Check sheet for the modelled part. Datum: model origin and axes. Units: mm. A direction names the side the tool comes from. Give positions to 0.01 mm unless a question says otherwise; leave off trailing zeros. Write each loop counter-clockwise with the first axis right and the second up, starting at its lowest first coordinate (ties: lowest second). Pieces come first, ordered by that corner, then holes. Notation, with made-up numbers: M 76,41 L 117,41 A36 cw 117,77 Z; hole C -34,10.25 d8. An arc over 180 degrees is marked long. Use CSV: the item, a comma, the result in double quotes. Start each with the question number.
1. Cross-section at A-A, the plane x = 16. Enter the section's corners in (y, z).
2. Mould release check, pull along Z, two halves, no side actions. Record for faces 1 (the face through (0, -6, 8)), 2 (the face through (19.699, 5.803, 0.285)), 3 (the face through (14.4, 5.8, 3.07)): +Z half, -Z half, draft (parallel to the pull), parting line (faces both ways), or undercut.
3. Depth check by flat-ended pin: P1, Ø5, axis at x = 5.5, y = 1.5, coming from the -Z side; P2, Ø4, axis at x = 16, z = 3, coming from the -Y side. Enter the tip coordinate at first touch or a pass-through.
4. Scan lines: line 1 (Y direction, x = -4.5, z = 8.5); line 2 (Z direction, x = 16, y = 5.8); line 3 (Z direction, x = 2, y = -0.75). Record each from-to range of solid material in increasing order.
5. Cross-section at D-D, the plane x = 6.5. Enter the section's corners in (y, z), and give its area (3 significant figures).
6. Access from +Z, -Z, +X, -X, +Y, -Y to the whole of each face (thin tool, end or side, straight path). Record for faces 4 (the face through (0, 0, 15.6)), 5 (the face through (-19.715, 5.803, 0.301)).
7. Cross-section at C-C, the plane z = 11. Enter the section's corners in (x, y), and give its area (3 significant figures).
8. Cross-section at B-B, the plane z = 3. Enter the section's corners in (x, y), and give its area (3 significant figures).
from build123d import *

# Parameters (mm, degrees)
SKETCH1_W           = 40
SKETCH1_H           = 12
BOSS_EXTRUDE1_DEPTH = 16
SKETCH2_R           = 1.6
SKETCH2_W           = 12
SKETCH2_H           = 0.6
CUT_EXTRUDE1_DEPTH  = 13
SKETCH3_W           = 15.6
SKETCH3_H           = 11.2
CUT_EXTRUDE2_DEPTH  = 41
FILLET1_R           = 1


with BuildPart() as part:
    # Sketch1 → Boss-Extrude1 (new body)
    with BuildSketch(Plane.XY):
        Rectangle(SKETCH1_W, SKETCH1_H)
    extrude(amount=BOSS_EXTRUDE1_DEPTH)

    # Sketch2 → Cut-Extrude1 (cut, through all)
    with BuildSketch(Plane.XZ.offset(6)):
        with Locations((-16, 3)):
            Circle(SKETCH2_R)
        with Locations((16, 3)):
            Circle(SKETCH2_R)
        with Locations((0, 4.8)):
            Rectangle(SKETCH2_W, SKETCH2_H)
    extrude(amount=-CUT_EXTRUDE1_DEPTH, mode=Mode.SUBTRACT)

    # Sketch3 → Cut-Extrude2 (cut, through all)
    with BuildSketch(Plane(origin=(20, 0, 0), x_dir=(0, 0, -1), z_dir=(1, 0, 0))):
        with Locations((-7.8, 0)):
            Rectangle(SKETCH3_W, SKETCH3_H)
    extrude(amount=-CUT_EXTRUDE2_DEPTH, mode=Mode.SUBTRACT)

    # Fillet1
    fillet1_edges = [part.edges().sort_by_distance(p)[0] for p in [
        (20, 5.8, 0),
        (-20, -5.8, 0),
        (-20, 5.8, 0),
        (20, -5.8, 0),
    ]]
    fillet(fillet1_edges, radius=FILLET1_R)


solid = part.part
Worked answers:
1,outline,"M -6,0 L -5.6,0 L -5.6,1.4 L -6,1.4 Z; M -6,4.6 L -5.6,4.6 L -5.6,15.6 L 5.6,15.6 L 5.6,4.6 L 6,4.6 L 6,16 L -6,16 Z; M 5.6,0 L 6,0 L 6,1.4 L 5.6,1.4 Z"
2,face 1,"draft"
2,face 2,"-Z half"
2,face 3,"undercut"
3,P1,"stops at z = 15.6"
3,P2,"stops at y = -6"
4,line 1,"y = -6 to -5.6, 5.6 to 6"
4,line 2,"z = 0 to 1.4, 4.6 to 16"
4,line 3,"z = 15.6 to 16"
5,outline,"M -6,0 L -5.6,0 L -5.6,15.6 L 5.6,15.6 L 5.6,0 L 6,0 L 6,16 L -6,16 Z"
5,area,"17.3 mm^2"
6,face 4,"-Z, +X, -X"
6,face 5,"-Z, -X, +Y, -Y"
7,outline,"M -20,-6 L 20,-6 L 20,-5.6 L -20,-5.6 Z; M -20,5.6 L 20,5.6 L 20,6 L -20,6 Z"
7,area,"32.0 mm^2"
8,outline,"M -20,-6 L -17.6,-6 L -17.6,-5.6 L -20,-5.6 Z; M -20,5.6 L -17.6,5.6 L -17.6,6 L -20,6 Z; M -14.4,-6 L 14.4,-6 L 14.4,-5.6 L -14.4,-5.6 Z; M -14.4,5.6 L 14.4,5.6 L 14.4,6 L -14.4,6 Z; M 17.6,-6 L 20,-6 L 20,-5.6 L 17.6,-5.6 Z; M 17.6,5.6 L 20,5.6 L 20,6 L 17.6,6 Z"
8,area,"26.9 mm^2"
